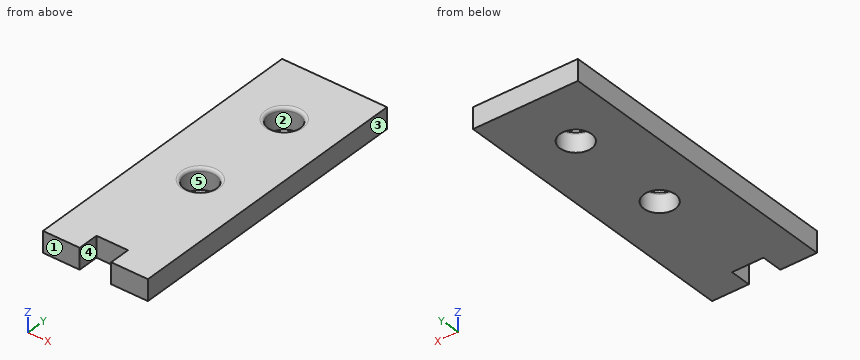
Autodesk Inventor part; units mm, degrees
ref_plane "YZ Plane" through (0, 0, 0) normal (1, 0, 0) x (0, 1, 0)
ref_plane "XZ Plane" through (0, 0, 0) normal (0, 1, 0) x (-1, 0, 0)
ref_plane "XY Plane" through (0, 0, 0) normal (0, 0, 1) x (1, 0, 0)
sketch "Sketch1" plane through (0, 0, 0) normal (0, 0, 1) x (1, 0, 0)
  line L0 (0, 0) -> (100, 0)
  line L1 (100, 0) -> (100, 285)
  line L2 (100, 285) -> (0, 285)
  line L3 (0, 285) -> (0, 0)
  dimension "d0" = 100
  dimension "d1" = 285
extrude "Extrusion1" add sketch "Sketch1" along normal blind 20
sketch "Sketch2" plane through (0, 0, 0) normal (0, 0, -1) x (-1, 0, 0)
  circle A0 centre (-50, 125) radius 15
  circle A1 centre (-50, 225) radius 15
  line L0 (0, 285) -> (0, 0)
  line L1 (0, 0) -> (-100, 0)
  line L2 (-100, 285) -> (0, 285)
  dimension "d5" = 30
  dimension "d6" = 50
  dimension "d7" = 50
  dimension "d9" = 100
  dimension "d17" = 60
extrude "Extrusion2" cut sketch "Sketch2" against normal up to next
sketch "Sketch3" plane through (0, 0, 0) normal (0, 0, -1) x (-1, 0, 0)
  line L0 (0, 0) -> (-100, 0)
  line L1 (-35, 0) -> (-35, 20)
  line L2 (-35, 20) -> (-65, 20)
  line L3 (-65, 20) -> (-65, 0)
  line L4 (0, 285) -> (0, 0)
  dimension "d12" = 20
  dimension "d13" = 30
  dimension "d14" = 35
extrude "Extrusion3" cut sketch "Sketch3" against normal up to next
sketch "Sketch4" plane through (0, 0, 0) normal (-1, 0, 0) x (0, 0, 1)
  line L0 (0, 285) -> (0, 0)
  line L1 (0, 0) -> (20, 0)
  line L2 (20, 285) -> (20, 0)
  line L3 (0, 285) -> (20, 285)
  line L4 (20, 285) -> (90.7107, 214.2893) construction
  line L5 (20, 285) -> (120, 285) construction
  dimension "d18" = 100
  dimension "d19" = 45
fillet "Fillet3" radius 3 2 edges at (65, 125, 20) (65, 225, 20)
properties part number "EndaHaldarar" material "Wood (Birch)"
The model under review builds one solid part; all positions refer to its coordinate system, in mm. Face numbers are marked on the shaded views. A direction names the side the tool comes from. Coordinates: 2 decimals unless noted, no trailing zeros. Write each loop counter-clockwise with the first axis right and the second up, starting at its lowest first coordinate (ties: lowest second). Pieces come first, ordered by that corner, then holes. Notation, with made-up numbers: (73, 32.5) - (114, 32.5) arc R22 cw to (114, 70.5) - close; hole circle Ø4 at (20, 11). An arc over 180 degrees is marked (long way). Write item = value, one per line.
(1) Machinability: for the marked faces 4 and 5, which of the approach directions +Z, -Z, +X, -X, +Y, -Y give a long, thin tool a straight path to every point of the face, cutting with its end or side? Answer none if there is none.
Result sheet:
face_4 = +Z, -Z, -Y
face_5 = +Z, -Z
(2) Consider section A-A, the plane y = 225. Give the boundary of the cut face in (x, z).
Result sheet:
outline = (0, 0) - (35, 0) - (35, 17) arc R3 ccw to (32, 20) - (0, 20) - close; (65, 0) - (100, 0) - (100, 20) - (68, 20) arc R3 ccw to (65, 17) - close
(3) Consider section B-B, the plane z = 3.75. Give the boundary of the cut face in (x, y), then the cut area to 3 significant figures.
Result sheet:
outline = (0, 0) - (35, 0) - (35, 20) - (65, 20) - (65, 0) - (100, 0) - (100, 285) - (0, 285) - close; hole circle Ø30 at (50, 125); hole circle Ø30 at (50, 225)
area = 26,500 mm^2
(4) For line 1 (Y direction, x = 50, z = 13.5); line 2 (X direction, y = 214, z = 15); line 3 (X direction, y = 233, z = 5), list the stretches that pass through material, from the lowest coordinate up. Write a range as [from, to].
Result sheet:
line_1 = [20, 110], [140, 210], [240, 285]
line_2 = [0, 39.8], [60.2, 100]
line_3 = [0, 37.31], [62.69, 100]
(5) Mouldability with a two-part tool opening along Y and no side actions: class the marked faces 1, 2 and 3 as pulls with the +Y half, pulls with the -Y half, needs draft (parallel to the pull), parting line crosses it, or undercut.
Result sheet:
face_1 = pulls with the -Y half
face_2 = undercut
face_3 = needs draft
(6) Consider section C-C, the plane x = 50. Give the boundary of the cut face in (y, z).
Result sheet:
outline = (20, 0) - (110, 0) - (110, 17) arc R3 ccw to (107, 20) - (20, 20) - close; (140, 0) - (210, 0) - (210, 17) arc R3 ccw to (207, 20) - (143, 20) arc R3 ccw to (140, 17) - close; (240, 0) - (285, 0) - (285, 20) - (243, 20) arc R3 ccw to (240, 17) - close
(7) For P1, Ø10, axis at x = 52, z = 7, coming from the -Y side; P2, Ø24, axis at x = 50, y = 225, coming from the -Z side, all flat-tipped, find the tip position at first contact; note any pin that passes through.
Result sheet:
P1 = 20
P2 = through
